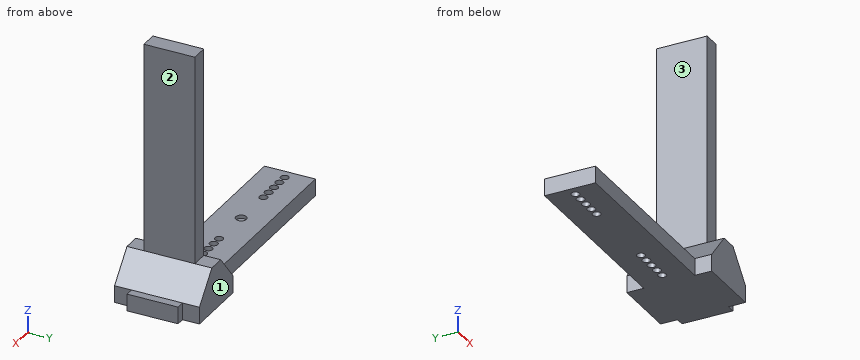
from build123d import *

# Parameters (mm, degrees)
SKETCH1_W           = 55
SKETCH1_H           = 15
SKETCH1_R           = 1.2
SKETCH1_W_2         = 22.5
BOSS_EXTRUDE1_DEPTH = 5
SKETCH2_R           = 1.577401702
CUT_EXTRUDE1_DEPTH  = 1
SKETCH2_3_W         = 5
SKETCH2_3_H         = 15
BOSS_EXTRUDE2_DEPTH = 70
BOSS_EXTRUDE3_DEPTH = 15
BOSS_EXTRUDE4_DEPTH = 5


with BuildPart() as part:
    # Sketch1 → Boss-Extrude1 (new body)
    with BuildSketch(Plane.XY):
        Rectangle(SKETCH1_W, SKETCH1_H)
        with Locations((-15.5, 0)):
            Circle(SKETCH1_R, mode=Mode.SUBTRACT)
        with Locations((-21.5, 0)):
            Circle(SKETCH1_R, mode=Mode.SUBTRACT)
        with Locations((24.5, 0)):
            Circle(SKETCH1_R, mode=Mode.SUBTRACT)
        with Locations((21.5, 0)):
            Circle(SKETCH1_R, mode=Mode.SUBTRACT)
        with Locations((18.5, 0)):
            Circle(SKETCH1_R, mode=Mode.SUBTRACT)
        with Locations((15.5, 0)):
            Circle(SKETCH1_R, mode=Mode.SUBTRACT)
        with Locations((12.5, 0)):
            Circle(SKETCH1_R, mode=Mode.SUBTRACT)
        with Locations((-24.5, 0)):
            Circle(SKETCH1_R, mode=Mode.SUBTRACT)
        with Locations((-18.5, 0)):
            Circle(SKETCH1_R, mode=Mode.SUBTRACT)
        with Locations((-12.5, 0)):
            Circle(SKETCH1_R, mode=Mode.SUBTRACT)
        with Locations((38.75, 0)):
            Rectangle(SKETCH1_W_2, SKETCH1_H)
    extrude(amount=BOSS_EXTRUDE1_DEPTH)

    # Sketch2 → Cut-Extrude1 (cut)
    with BuildSketch(Plane.XY.offset(5)):
        Circle(SKETCH2_R)
    extrude(amount=-CUT_EXTRUDE1_DEPTH, mode=Mode.SUBTRACT)

    # Sketch2<3> → Boss-Extrude2 (add)
    with BuildSketch(Plane.XY.offset(5)):
        with Locations((38, 0)):
            Rectangle(SKETCH2_3_W, SKETCH2_3_H)
    extrude(amount=BOSS_EXTRUDE2_DEPTH)

    # Sketch6 → Boss-Extrude3 (add)
    with BuildSketch(Plane(origin=(0, 7.5, 0), x_dir=(1, 0, 0), z_dir=(0, 1, 0))):
        Polygon((28.5, -5), (35.5, -13.282174024), (35.5, -5), align=None)
    boss_extrude3 = extrude(amount=-BOSS_EXTRUDE3_DEPTH)

    # Mirror1: Boss-Extrude3 across plane
    add(boss_extrude3.mirror(Plane(origin=(38, 0, 0), x_dir=(0, 0, 1), z_dir=(1, 0, 0))))

    # Sketch7 → Boss-Extrude4 (add)
    with BuildSketch(Plane(origin=(0, 7.5, 0), x_dir=(1, 0, 0), z_dir=(0, 1, 0))):
        Polygon((35.5, -13.282174024), (28.5, -5), (28.5, 0), (47.5, 0), (47.5, -5), (40.5, -13.282174024), align=None)
    boss_extrude4 = extrude(amount=BOSS_EXTRUDE4_DEPTH)

    # Mirror2: Boss-Extrude4 across plane
    add(boss_extrude4.mirror(Plane(origin=(0, 0, 0), x_dir=(0, 0, 1), z_dir=(0, -1, 0))))


solid = part.part
Input: part model. Units: mm. Frame: model coordinates. Face numbers are marked on the shaded views. A direction names the side the tool comes from. Coordinates: 2 decimals unless noted, no trailing zeros. Loops run counter-clockwise (first coordinate to the right, second up) from the corner with the lowest first, then second, coordinate; pieces in that order, holes last.
(1) Section B-B on y = 6.5. Return the cut outline in (x, z).
(2) Material intervals for probe 1 along Y at (x, z) = (15.5, 2.55); probe 2 along Y at (x, z) = (0, 4.6); probe 3 along X at (y, z) = (4, 44), sorted ascending.
(3) Section A-A on x = 21.5. Return the cut outline in (y, z), then the cut area to 3 significant figures.
(4) Section D-D on y = 0. Count the separate pieces of the cut face and the enclosed holes in it, then the cut area to 3 significant figures.
(5) Set-up query: the marked faces 1, 2 and 3. Return all of +Z, -Z, +X, -X, +Y, -Y with unobstructed straight access to the full face (end or side cutting, diameter ignored); none if empty.
(6) First-contact query: pin 1 Ø4.5 at (x, y) = (-7, 0) entering from +Z; pin 2 Ø3 at (x, y) = (12.5, 0) entering from -Z; pin 3 Ø1.9 at (x, y) = (21.5, 0) entering from +Z; pin 4 Ø5.5 at (x, z) = (38.5, 41.5) entering from +Y. Flat tips, straight axial feed; report the tip coordinate or a pass-through.
(7) Section C-C on z = 52. Return the cut outline in (x, y), then the cut area to 3 significant figures.
Data:
1. outline: (-27.5, 0) - (50, 0) - (50, 5) - (47.5, 5) - (40.5, 13.28) - (40.5, 75) - (35.5, 75) - (35.5, 13.28) - (28.5, 5) - (-27.5, 5) - close
2. probe 1: y = -7.5 to -1.2, 1.2 to 7.5
2. probe 2: y = -7.5 to -1.58, 1.58 to 7.5
2. probe 3: x = 35.5 to 40.5
3. outline: (-7.5, 0) - (-1.2, 0) - (-1.2, 5) - (-7.5, 5) - close; (1.2, 0) - (7.5, 0) - (7.5, 5) - (1.2, 5) - close
3. area: 63.0 mm2
4. separate pieces: 11
4. enclosed holes: 0
4. area: 672 mm2
5. face 1: +Z, -Z, +X, -X, +Y
5. face 2: +Z, +X, +Y, -Y
5. face 3: +Z, -X, +Y, -Y
6. pin 1: stops at z = 5
6. pin 2: stops at z = 0
6. pin 3: passes through
6. pin 4: stops at y = 7.5
7. outline: (35.5, -7.5) - (40.5, -7.5) - (40.5, 7.5) - (35.5, 7.5) - close
7. area: 75.0 mm2
